```python
from build123d import *

# Parameters (mm, degrees)
SKETCH_1_W             = 160
SKETCH_1_H             = 100
EXTRUDE_1_DEPTH        = 1.6
FILLET_1_R             = 3
HOLE_WIZARD_M3_1_D     = 4.4
HOLE_WIZARD_M3_1_DEPTH = 6


with BuildPart() as part:
    # ｽｹｯﾁ1 → ﾎﾞｽ - 押し出し1 (new body)
    with BuildSketch(Plane.XY):
        Rectangle(SKETCH_1_W, SKETCH_1_H)
    extrude(amount=EXTRUDE_1_DEPTH)

    # ﾌｨﾚｯﾄ1
    fillet_1_edges = [part.edges().sort_by_distance(p)[0] for p in [
        (-80, 50, 0.8),
        (80, 50, 0.8),
        (80, -50, 0.8),
        (-80, -50, 0.8),
    ]]
    fillet(fillet_1_edges, radius=FILLET_1_R)

    # M3 すきま穴1
    with Locations(Plane.XY.offset(1.6)):
        with Locations((-75, -45), (-75, 45), (75, 45), (75, -45)):
            Hole(HOLE_WIZARD_M3_1_D / 2, depth=HOLE_WIZARD_M3_1_DEPTH)


solid = part.part
```
Geometry check sheet. Reference: the model listing, model coordinates, mm. Coordinates: 2 decimals unless noted, no trailing zeros. Write each loop counter-clockwise with the first axis right and the second up, starting at its lowest first coordinate (ties: lowest second). Pieces come first, ordered by that corner, then holes. Notation, with made-up numbers: M 23.25,20 L 56.25,20 A6 cw 56.25,29 Z; hole C -2,8.25 d5. An arc over 180 degrees is marked long. Use one line per item in the form item = value. Start each with the question number.
1) Go/stop test with a flat-tipped pin: pin 1 Ø4 at (x, y) = (75, 45) entering from +Z. Record where the tip stops, or that it passes through.
2) Section check A-A on x = 75. Enter the section's corners in (y, z).
3) Release check for a two-part mould opening along Y. For faces 1 (the flat face through (-1, 1, 1.6)), 2 (the cylindrical face through (-79.14, 49.1, 0.81)), 3 (the cylindrical face through (-76.02, -46.95, 0.79)) record: pulls with the +Y half, pulls with the -Y half, needs draft (parallel to the pull), parting line crosses it, or undercut.
4) Section check B-B on y = 45. Enter the section's corners in (x, z), and give its area (3 significant figures).
5) Thickness scan on probe 1 along Y at (x, z) = (75, 0.85). Record the ranges inside material, lowest first. Write a range as from..to.
Responses:
q1.pin_1 = through
q2.outline = M -50,0 L -47.2,0 L -47.2,1.6 L -50,1.6 Z; M -42.8,0 L 42.8,0 L 42.8,1.6 L -42.8,1.6 Z; M 47.2,0 L 50,0 L 50,1.6 L 47.2,1.6 Z
q3.face_1 = needs draft
q3.face_2 = pulls with the +Y half
q3.face_3 = undercut
q4.outline = M -80,0 L -77.2,0 L -77.2,1.6 L -80,1.6 Z; M -72.8,0 L 72.8,0 L 72.8,1.6 L -72.8,1.6 Z; M 77.2,0 L 80,0 L 80,1.6 L 77.2,1.6 Z
q4.area = 242 mm2
q5.probe_1 = -50..-47.2, -42.8..42.8, 47.2..50
